from build123d import *

# Parameters (mm, degrees)
F0_W     = 311.15
F0_H     = 438.15
F1_DEPTH = 9.525
F2_W     = 311.15
F2_H     = 19.05
F3_DEPTH = 6.35


with BuildPart() as f1:
    # F0 (on Front) → F1 (new body, symmetric)
    with BuildSketch(Plane.XZ):
        with Locations((-92.3289953259, 219.075)):
            Rectangle(F0_W, F0_H)
        with Locations((-92.3289953259, -219.075)):
            Rectangle(F0_W, F0_H)
    extrude(amount=F1_DEPTH, both=True)

    # F2 (on face) → F3 (cut)
    with BuildSketch(Plane(origin=(0, 9.525, 0), x_dir=(-1, 0, 0), z_dir=(0, 1, 0))):
        with Locations((92.3289953259, 309.5625)):
            Rectangle(F2_W, F2_H)
    extrude(amount=-F3_DEPTH, mode=Mode.SUBTRACT)


solid = f1.part
Source: CAD feature listing. Evaluate the final solid. Frame: model axes, mm. Give positions to 0.01 mm unless a question says otherwise; leave off trailing zeros. Return JSON: item names as keys, results as strings. Group by question number.
1) Pin query (flat end, axial travel): P1, Ø15, axis at x = -132.5, z = 310, coming from the +Y side (3 decimals). Return the tip coordinate at first contact, or that it passes through.
2) Material intervals for line 1 along Z through (x, y) = (-29.5, 5), sorted ascending. Write a range as [from, to].
3) Pull-direction query (Z, two-part tool) for faces 1 (the face through (-90, 3.175, 310)), 2 (the face through (-95, 9.525, -64)), 3 (the face through (-95, 0, 438.15)); classes: pulls with the +Z half, pulls with the -Z half, needs draft (parallel to the pull), parting line crosses it, or undercut.
Recorded:
{
 "1": {"P1": "stops at y = 3.175"},
 "2": {"line 1": "z = [-438.15, 300.04], [319.09, 438.15]"},
 "3": {"face 1": "undercut", "face 2": "needs draft", "face 3": "pulls with the +Z half"}
}
